Geometry check sheet. Reference: the model listing, model coordinates, mm. Face numbers are marked on the shaded views. A direction names the side the tool comes from. Give positions to 0.01 mm unless a question says otherwise; leave off trailing zeros. Order: outer loops, then holes, each group sorted by start corner. A loop starts at its lowest first (then second) coordinate and runs counter-clockwise, first axis right, second up. Notation, with made-up numbers: M 9,5 L 49,5 A17 ccw 49,24 Z; hole C 34.25,44 d9. An arc over 180 degrees is marked long. Answer as a JSON object with one key per item and string values. Group by question number.
from build123d import *

# Parameters (mm, degrees)
SKETCH3_R           = 0.4
BOSS_EXTRUDE1_DEPTH = 5


with BuildPart() as part:
    # Sketch1 → Revolve1 (revolve)
    with BuildSketch(Plane(origin=(0, 0, 0), x_dir=(0, 0, -1), z_dir=(1, 0, 0))):
        with BuildLine():
            Line((-4.25, 7.3), (-4.25, 5.049389861))
            ThreePointArc((-4.25, 5.049389861), (-4.249388291, 5.024664681), (-4.247554662, 5))
            ThreePointArc((-4.247554662, 5), (-4, 0), (-4.247554662, -5))
            ThreePointArc((-4.247554662, -5), (-4.249388291, -5.024664681), (-4.25, -5.049389861))
            Line((-4.25, -5.049389861), (-4.25, -7.3))
            ThreePointArc((-4.25, -7.3), (-4.103553391, -7.653553391), (-3.75, -7.8))
            Line((-3.75, -7.8), (-2.75, -7.8))
            Line((-2.75, -7.8), (-2.75, -7))
            Line((-2.75, -7), (0, -7))
            Line((0, -7), (0, 7))
            Line((0, 7), (-2.75, 7))
            Line((-2.75, 7), (-2.75, 7.8))
            Line((-2.75, 7.8), (-3.75, 7.8))
            ThreePointArc((-3.75, 7.8), (-4.103553391, 7.653553391), (-4.25, 7.3))
        make_face()
    revolve(axis=Axis((0, 12.565257793, 0), (0, -1, 0)))

    # Sketch3 → Boss-Extrude1 (add)
    with BuildSketch(Plane.XZ.offset(7)):
        with Locations(Location((-2.825, 0, 0), (0, 0, 75.178560111))):
            Circle(SKETCH3_R)
        with Locations(Location((2.825, 0, 0), (0, 0, 90))):
            Circle(SKETCH3_R)
    extrude(amount=BOSS_EXTRUDE1_DEPTH)


solid = part.part
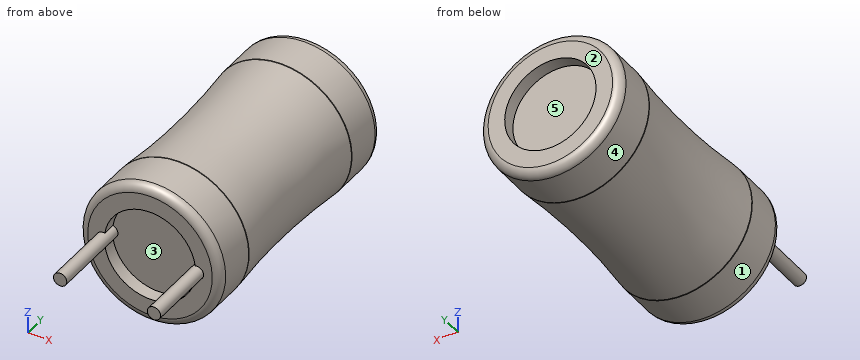
1. Cross-section at A-A (z = 0). Record the cut outline in (x, y) (3 decimals), and give its area (3 significant figures).
2. Depth check by flat-ended pin: pin 1 (1 mm diameter, centred on x = 2.5, y = 4.5, fed in from +Z); pin 2 (4 mm diameter, centred on y = -2.5, z = 3.5, fed in from +X); pin 3 (3 mm diameter, centred on y = 0, z = 2.5, fed in from +X). Enter the tip coordinate at first touch or a pass-through.
3. Release check for a two-part mould opening along Z. For the marked faces 1, 2 and 3 record: released by +Z, released by -Z, zero draft, split by the parting line, or undercut.
4. Cross-section at B-B (x = 0). Record the cut outline in (y, z).
5. Thickness scan on line 1 along Z through (x, y) = (0, 7.3); line 2 along Y through (x, z) = (0.25, -2). Record the ranges inside material, lowest first. Write a range as [from, to].
6. Cross-section at D-D (y = -5.25). Record the cut outline in (x, z), and give its area (3 significant figures).
7. Access from +Z, -Z, +X, -X, +Y, -Y to the whole of each face (thin tool, end or side, straight path). Record for the marked faces 4 and 5.
8. Cross-section at C-C (y = -9.5). Record the cut outline in (x, z) (3 decimals), and give its area (3 significant figures).
Report:
{
 "1": {"outline": "M -4.25,-7.3 A0.5 ccw -3.75,-7.8 L -3.225,-7.8 L -3.225,-12 L -2.425,-12 L -2.425,-7 L 2.425,-7 L 2.425,-12 L 3.225,-12 L 3.225,-7.8 L 3.75,-7.8 A0.5 ccw 4.25,-7.3 L 4.25,-5.049 A0.5 ccw 4.248,-5 A50.618 cw 4.248,5 A0.5 ccw 4.25,5.049 L 4.25,7.3 A0.5 ccw 3.75,7.8 L 2.75,7.8 L 2.75,7 L -2.75,7 L -2.75,7.8 L -3.75,7.8 A0.5 ccw -4.25,7.3 L -4.25,5.049 A0.5 ccw -4.248,5 A50.618 cw -4.248,-5 A0.5 ccw -4.25,-5.049 Z", "area": "127 mm2"},
 "2": {"pin 1": "stops at z = 3.7", "pin 2": "stops at x = 3.78", "pin 3": "stops at x = 3.87"},
 "3": {"face 1": "split by the parting line", "face 2": "zero draft", "face 3": "undercut"},
 "4": {"outline": "M -7.8,-3.75 A0.5 ccw -7.3,-4.25 L -5.05,-4.25 A0.5 ccw -5,-4.25 A50.62 cw 5,-4.25 A0.5 ccw 5.05,-4.25 L 7.3,-4.25 A0.5 ccw 7.8,-3.75 L 7.8,-2.75 L 7,-2.75 L 7,2.75 L 7.8,2.75 L 7.8,3.75 A0.5 ccw 7.3,4.25 L 5.05,4.25 A0.5 ccw 5,4.25 A50.62 cw -5,4.25 A0.5 ccw -5.05,4.25 L -7.3,4.25 A0.5 ccw -7.8,3.75 L -7.8,2.75 L -7,2.75 L -7,-2.75 L -7.8,-2.75 Z"},
 "5": {"line 1": "z = [-4.25, -2.75], [2.75, 4.25]", "line 2": "y = [-7, 7]"},
 "6": {"outline": "C 0,0 d8.5", "area": "56.7 mm2"},
 "7": {"face 4": "+Y, -Y", "face 5": "+Y"},
 "8": {"outline": "C -2.825,0 d0.8; C 2.825,0 d0.8", "area": "1.01 mm2"}
}
